Read the model definition and answer for the solid it produces. Units are mm, in the model's axes. A direction names the side the tool comes from. Coordinates: 2 decimals unless noted, no trailing zeros. Write each loop counter-clockwise with the first axis right and the second up, starting at its lowest first coordinate (ties: lowest second). Pieces come first, ordered by that corner, then holes.
(1) Given pin 1 (3 mm diameter, centred on y = -39, z = -28, fed in from -X); pin 2 (1.8 mm diameter, centred on x = -48.5, z = -16.5, fed in from -Y); pin 3 (2.5 mm diameter, centred on x = 37, z = 3, fed in from -Y); pin 4 (1.1 mm diameter, centred on y = -36, z = 3, fed in from +X), each flat-ended and moving along its own axis, determine where each tip first touches the part or whether it passes through.
(2) Which of the six approach directions +Z, -Z, +X, -X, +Y, -Y give full straight-line access (tool end or side, diameter ignored) to faces 4 (the cylindrical face through (-24.36, -41.73, -25.34)), 5 (the flat face through (0, -36.5, 2)), 6 (the flat face through (39, -36.5, 2))?
(3) Determine the mould class of faces 1 (the flat face through (-31.75, -42, -22)), 2 (the flat face through (-1, 1, 0)), 3 (the cylindrical face through (18.89, 46.778, -27.985)) for opening direction Y: pulls with the +Y half, pulls with the -Y half, needs draft (parallel to the pull), parting line crosses it, or undercut.
(4) The part is cut by section B-B, the plane z = -20.5. Determine the outline of the cut face in (x, y), and give its area (3 significant figures).
(5) The part is cut by section C-C, the plane y = -18. Determine the outline of the cut face in (x, z).
(6) The part is cut by section D-D, the plane x = -27.5. Determine the outline of the cut face in (y, z), and give its area (3 significant figures).
(7) Straight lines are drawn through the part: line 1 along X through (y, z) = (1.5, -11); line 2 along Z through (x, y) = (-43.5, -9); line 3 along Z through (x, y) = (-11, 32.5). For each, find the intervals that lie inside material, in ascending order.
(8) The part is cut by section A-A, the plane x = 30. Determine the outline of the cut face in (y, z).
```python
from build123d import *

# Parameters (mm, degrees)
SKETCH1_W           = 93.5
SKETCH1_H           = 73
BOSS_EXTRUDE1_DEPTH = 5
BOSS_EXTRUDE3_START = -18
BOSS_EXTRUDE3_DEPTH = 20
SKETCH3_W           = 40
SKETCH3_H           = 72
BOSS_EXTRUDE4_DEPTH = 5
FILLET2_R           = 1
BOSS_EXTRUDE5_START = -15
BOSS_EXTRUDE5_DEPTH = 15


with BuildPart() as part:
    # Sketch1 → Boss-Extrude1 (new body)
    with BuildSketch(Plane.XY):
        Rectangle(SKETCH1_W, SKETCH1_H)
    extrude(amount=BOSS_EXTRUDE1_DEPTH)

    # Sketch2 → Boss-Extrude3 (add)
    with BuildSketch(Plane(origin=(46.75, 0, 0), x_dir=(0, 0, -1), z_dir=(1, 0, 0)).offset(BOSS_EXTRUDE3_START)):
        with BuildLine():
            ThreePointArc((-2.434820811, 39.673585924), (-3.782270226, 38.139218536), (-5, 36.5))
            Line((-5, 36.5), (0, 36.5))
            Line((0, 36.5), (0, 36.002201306))
            ThreePointArc((0, 36.002201306), (0.106466288, 36.451197416), (0.403195013, 36.804587627))
            ThreePointArc((0.403195013, 36.804587627), (24.169553289, 43.313947092), (46.060330973, 32))
            Line((46.060330973, 32), (39.766102339, 28.366025404))
            ThreePointArc((39.766102339, 28.366025404), (39.300176512, 27.241180955), (40.266102339, 26.5))
            Line((40.266102339, 26.5), (49.466267311, 26.5))
            ThreePointArc((49.466267311, 26.5), (49.981952839, 26.567626217), (50.462764505, 26.765931563))
            Line((50.462764505, 26.765931563), (52.589346112, 27.987989793))
            ThreePointArc((52.589346112, 27.987989793), (53.05994511, 28.607366306), (52.944303456, 29.376598189))
            ThreePointArc((52.944303456, 29.376598189), (27.548560845, 46.861682099), (-2.434820811, 39.673585924))
        make_face()
    boss_extrude3 = extrude(amount=-BOSS_EXTRUDE3_DEPTH)

    # Mirror1: Boss-Extrude3 across plane
    add(boss_extrude3.mirror(Plane(origin=(0, 0, 0), x_dir=(0, 0, 1), z_dir=(1, 0, 0))))

    # Sketch3 → Boss-Extrude4 (add)
    with BuildSketch(Plane(origin=(46.75, 0, 0), x_dir=(0, 0, -1), z_dir=(1, 0, 0))):
        with Locations((15, 0.5)):
            Rectangle(SKETCH3_W, SKETCH3_H)
    boss_extrude4 = extrude(amount=BOSS_EXTRUDE4_DEPTH)

    # Mirror3: Boss-Extrude4 across plane
    add(boss_extrude4.mirror(Plane(origin=(0, 0, 0), x_dir=(0, 0, 1), z_dir=(1, 0, 0))))

    # Fillet2
    fillet2_edges = [part.edges().sort_by_distance(p)[0] for p in [
        (-46.75, 0.5, 0),
        (46.75, 0.5, 0),
        (46.75, 0.5, -35),
        (-46.75, 0.5, -35),
    ]]
    fillet(fillet2_edges, radius=FILLET2_R)

    # Sketch2_5 → Boss-Extrude5 (add)
    with BuildSketch(Plane(origin=(46.75, 0, 0), x_dir=(0, 0, -1), z_dir=(1, 0, 0)).offset(BOSS_EXTRUDE5_START)):
        with BuildLine():
            ThreePointArc((0.403195013, -36.804587627), (0.106466288, -36.451197416), (0, -36.002201306))
            Line((0, -36.002201306), (-5, -36.5))
            ThreePointArc((-5, -36.5), (-3.782270226, -38.139218536), (-2.434820811, -39.673585924))
            ThreePointArc((-2.434820811, -39.673585924), (23.559962361, -44.796829736), (50, -46.5))
            Line((50, -46.5), (50, -43.5))
            ThreePointArc((50, -43.5), (24.995023445, -41.682507765), (0.403195013, -36.804587627))
        make_face()
    boss_extrude5 = extrude(amount=-BOSS_EXTRUDE5_DEPTH)

    # Mirror4: Boss-Extrude5 across plane
    add(boss_extrude5.mirror(Plane(origin=(0, 0, 0), x_dir=(0, 0, 1), z_dir=(1, 0, 0))))


solid = part.part
```
Computed:
1. pin 1: passes through
1. pin 2: stops at y = -35.5
1. pin 3: stops at y = -36.5
1. pin 4: stops at x = 51.75
2. face 4: -Z, +X, -X
2. face 5: +Z, -Z, -Y
2. face 6: +Z, -Z, +X, -Y
3. face 1: needs draft
3. face 2: undercut
3. face 3: pulls with the +Y half
4. outline: (-51.75, -35.5) - (-46.75, -35.5) - (-46.75, 36.5) - (-51.75, 36.5) - close; (-31.75, -44.37) - (-16.75, -44.37) - (-16.75, -41.02) - (-31.75, -41.02) - close; (-28.75, 43.5) - (-8.75, 43.5) - (-8.75, 47.5) - (-28.75, 47.5) - close; (8.75, 43.5) - (28.75, 43.5) - (28.75, 47.5) - (8.75, 47.5) - close; (16.75, -44.37) - (31.75, -44.37) - (31.75, -41.02) - (16.75, -41.02) - close; (46.75, -35.5) - (51.75, -35.5) - (51.75, 36.5) - (46.75, 36.5) - close
4. area: 981 mm2
5. outline: (-51.75, -35) - (-47.75, -35) arc R1 ccw to (-46.75, -34) - (-46.75, -1) arc R1 cw to (-45.75, 0) - (45.75, 0) arc R1 cw to (46.75, -1) - (46.75, -34) arc R1 ccw to (47.75, -35) - (51.75, -35) - (51.75, 5) - (-51.75, 5) - close
6. outline: (-46.5, -50) - (-43.5, -50) arc R203.53 cw to (-36.8, -0.4) arc R1 cw to (-36, 0) - (36, 0) arc R1 cw to (36.8, -0.4) arc R33.88 cw to (32, -46.06) - (28.37, -39.77) arc R1 ccw to (26.5, -40.27) - (26.5, -49.47) arc R2 ccw to (26.77, -50.46) - (27.99, -52.59) arc R1 ccw to (29.38, -52.94) arc R37.88 ccw to (39.67, 2.43) arc R25 ccw to (36.5, 5) - (-36.5, 5) arc R25 ccw to (-39.67, 2.43) arc R203.53 ccw to start
6. area: 831 mm2
7. line 1: x = -51.75 to -46.75, 46.75 to 51.75
7. line 2: z = 0 to 5
7. line 3: z = -50.81 to -45.61, 0 to 5
8. outline: (-46.5, -50) - (-43.5, -50) arc R203.53 cw to (-36.8, -0.4) arc R1 cw to (-36, 0) - (36.5, 0) - (36.5, 5) - (-36.5, 5) arc R25 ccw to (-39.67, 2.43) arc R203.53 ccw to start
